Autodesk Inventor part; units mm, degrees
ref_plane "YZ Plane" through (0, 0, 0) normal (1, 0, 0) x (0, 1, 0)
ref_plane "XZ Plane" through (0, 0, 0) normal (0, 1, 0) x (-1, 0, 0)
ref_plane "XY Plane" through (0, 0, 0) normal (0, 0, 1) x (1, 0, 0)
sketch "Sketch1" plane through (0, 0, 0) normal (0, 0, 1) x (1, 0, 0)
  circle A0 centre (0, 0) radius 19.685
  dimension "d0" = 39.37
extrude "Extrusion1" add sketch "Sketch1" along normal blind 25.4
fillet "Fillet1" radius 15.748 1 edges at (-19.685, 0, 25.4)
sketch "Sketch2" plane through (0, 0, 0) normal (0, 0, -1) x (-1, 0, 0)
  line L0 (-13.081, -13.081) -> (13.081, -13.081)
  line L1 (13.081, -13.081) -> (13.081, 13.081)
  line L2 (13.081, 13.081) -> (-13.081, 13.081)
  line L3 (-13.081, 13.081) -> (-13.081, -13.081)
  point P0 (0, 0)
  dimension "d4" = 26.162
  dimension "d5" = 26.162
  dimension "d6" = 13.081
  dimension "d8" = 13.081
extrude "Extrusion2" cut sketch "Sketch2" against normal blind 12.7
properties part number "SharpCap"
Model file for the job. Use its own axes, mm. A direction names the side the tool comes from. Coordinates: 2 decimals unless noted, no trailing zeros. Answer as CSV lines item,"result".
(1) Flat gauge pins, fed straight in: pin 1 (10 mm diameter, centred on x = -8, z = 15.5, fed in from -Y); pin 2 (4 mm diameter, centred on x = -4.5, z = 7.5, fed in from +Y); pin 3 (1 mm diameter, centred on y = -15, z = 6.5, fed in from -X). Where does each tip first touch, or does it go through?
Geometry says:
pin 1,"stops at y = -19.01"
pin 2,"stops at y = 19.53"
pin 3,"stops at x = -13.31"
(2) Wall check: line 1 along Y through (x, z) = (1, 11); line 2 along X through (y, z) = (13, 2.75); line 3 along Y through (x, z) = (0.5, 3). Give the ranges that are in metal, low to high.
Geometry says:
line 1,"y = -19.6 to -13.08, 13.08 to 19.6"
line 2,"x = -14.78 to -13.08, 13.08 to 14.78"
line 3,"y = -19.68 to -13.08, 13.08 to 19.68"
(3) 3-axis set-ups, long thin cutter, end or side, ignore diameter. For faces 4 (the flat face through (-15, 2, 0)), 5 (the flat face through (0, -13.081, 6)): which of +Z, -Z, +X, -X, +Y, -Y reach the whole face in a straight line?
Geometry says:
face 4,"-Z, +X, -X, +Y, -Y"
face 5,"-Z"
(4) Pull direction Y, two halves, no side cores. Call faces 1 (the flat face through (0, 0, 25.4)), 2 (the flat face through (13.081, 0, 6)), 3 (the cylindrical face through (-15.62, 11.98, 4.76)): +Y half, -Y half, draft (parallel to the pull), parting line (faces both ways), or undercut.
Geometry says:
face 1,"draft"
face 2,"undercut"
face 3,"parting line"
